The listing builds one solid part. Answer for the finished solid, in the listing's coordinates (mm). A direction names the side the tool comes from. Coordinates: 2 decimals unless noted, no trailing zeros. Order: outer loops, then holes, each group sorted by start corner. A loop starts at its lowest first (then second) coordinate and runs counter-clockwise, first axis right, second up.
Autodesk Inventor part; units mm, degrees
ref_plane "YZ Plane" through (0, 0, 0) normal (1, 0, 0) x (0, 1, 0)
ref_plane "XZ Plane" through (0, 0, 0) normal (0, 1, 0) x (-1, 0, 0)
ref_plane "XY Plane" through (0, 0, 0) normal (0, 0, 1) x (1, 0, 0)
sketch "Sketch_BoxBase" plane through (0, 0, 0) normal (0, 0, 1) x (1, 0, 0)
  line L0 (0, 56.7) -> (0, -56.7) construction
  line L1 (-53.9, 0) -> (53.9, 0) construction
  line L2 (-36.5, 38.5) -> (36.5, 38.5)
  line L3 (36.5, 38.5) -> (36.5, -38.5)
  line L4 (36.5, -38.5) -> (-36.5, -38.5)
  line L5 (-36.5, -38.5) -> (-36.5, 38.5)
  line L6 (-36.5, 38.5) -> (36.5, -38.5) construction
  line L7 (36.5, 38.5) -> (-36.5, -38.5) construction
  line L8 (-38.5, 40.5) -> (38.5, 40.5)
  line L9 (38.5, 40.5) -> (38.5, -40.5)
  line L10 (38.5, -40.5) -> (-38.5, -40.5)
  line L11 (-38.5, -40.5) -> (-38.5, 40.5)
  line L12 (-38.5, 40.5) -> (38.5, -40.5) construction
  line L13 (38.5, 40.5) -> (-38.5, -40.5) construction
  point P0 (0, 0)
  point P1 (-20, -33.5)
  point P2 (20, -33.5)
  dimension "d4" = 73
  dimension "d5" = 77
  dimension "d6" = 77
  dimension "d7" = 81
  dimension "d23" = 40
  dimension "d24" = 20
  dimension "d25" = 7
  dimension "d26" = 7
extrude "Extr_Edge" add sketch "Sketch_BoxBase" along normal blind 21
extrude "Extr_Bottom" add sketch "Sketch_BoxBase" along normal blind 3 contours L2 L3 L4 L5
hole "Hole2" at (-20, -33.5, 0) at (20, -33.5, 0) direction (0, 0, 1) diameter 4 end through all
fillet "Fillet1" radius 1 1 edges at (38.5, 40.5, 10.5)
fillet "Fillet2" radius 1 4 edges at (-38.5, 40.5, 10.5) (-38.5, -40.5, 10.5) (38.5, -40.5, 10.5) (-38.5, 0, 0)
properties part number "Enclosure"
1) Section C-C (z = 4.25) is taken. Give the vertices of the cut face in (x, y).
2) Determine the mould class of faces 3 (the face through (-1, 1, 3)), 4 (the face through (0, 1, 0)), 5 (the face through (-1, 40.5, 10)), 6 (the face through (1, -40.5, 10)) for opening direction Y: released by +Y, released by -Y, zero draft, split by the parting line, or undercut.
3) Section B-B (x = 20) is taken. Give the vertices of the cut face in (y, z), then the cut area to 3 significant figures.
4) Consider L1, parallel to X at y = -33.5, z = 2.1; L2, parallel to Y at x = 20, z = 1.95; L3, parallel to Y at x = 13.5, z = 10.5. Determine where each line is inside the solid, lowest interval first.
5) Section D-D (y = 13.5) is taken. Give the vertices of the cut face in (x, z), then the cut area to 3 significant figures.
6) Section A-A (y = -33.5) is taken. Give the vertices of the cut face in (x, z).
7) This flat-tipped pin is pushed along its axis until it touches: P1, Ø4, axis at x = 16, y = 27.5, coming from the +Z side. Where does it stop, or does it pass through?
8) A tool of negligible diameter and unlimited length cuts with its end or side. For faces 1 (the face through (-20.601, -31.592, 1.521)), 2 (the face through (-1, 38.5, 12)), from which of +Z, -Z, +X, -X, +Y, -Y can it reach the whole face along a straight path? Write none if from no direction.
Filled sheet:
1. outline: (-38.5, -39.5) arc R1 ccw to (-37.5, -40.5) - (37.5, -40.5) arc R1 ccw to (38.5, -39.5) - (38.5, 39.5) arc R1 ccw to (37.5, 40.5) - (-37.5, 40.5) arc R1 ccw to (-38.5, 39.5) - close; hole (-36.5, -38.5) - (36.5, -38.5) - (36.5, 38.5) - (-36.5, 38.5) - close
2. face 3: undercut
2. face 4: zero draft
2. face 5: released by +Y
2. face 6: released by -Y
3. outline: (-40.5, 0) - (-35.5, 0) - (-35.5, 3) - (-38.5, 3) - (-38.5, 21) - (-40.5, 21) - close; (-31.5, 0) - (40.5, 0) - (40.5, 21) - (38.5, 21) - (38.5, 3) - (-31.5, 3) - close
3. area: 303 mm2
4. L1: x = -38.5 to -22, -18 to 18, 22 to 38.5
4. L2: y = -40.5 to -35.5, -31.5 to 40.5
4. L3: y = -40.5 to -38.5, 38.5 to 40.5
5. outline: (-38.5, 1) arc R1 ccw to (-37.5, 0) - (38.5, 0) - (38.5, 21) - (36.5, 21) - (36.5, 3) - (-36.5, 3) - (-36.5, 21) - (-38.5, 21) - close
5. area: 303 mm2
6. outline: (-38.5, 1) arc R1 ccw to (-37.5, 0) - (-22, 0) - (-22, 3) - (-36.5, 3) - (-36.5, 21) - (-38.5, 21) - close; (-18, 0) - (18, 0) - (18, 3) - (-18, 3) - close; (22, 0) - (38.5, 0) - (38.5, 21) - (36.5, 21) - (36.5, 3) - (22, 3) - close
7. P1: stops at z = 3
8. face 1: +Z, -Z
8. face 2: +Z
